The drawing under review shows one solid part. Ordinate dimensions are in mm from its lowest x, y, z. Coordinates: 2 decimals unless noted, no trailing zeros. Loops run counter-clockwise (first coordinate to the right, second up) from the corner with the lowest first, then second, coordinate; pieces in that order, holes last. Notation, with made-up numbers: M -12,-38 L 8,-38 A8 cw 8,-29 Z; hole C 83.5,30.25 d2. An arc over 180 degrees is marked long. Use one line per item in the form item = value.
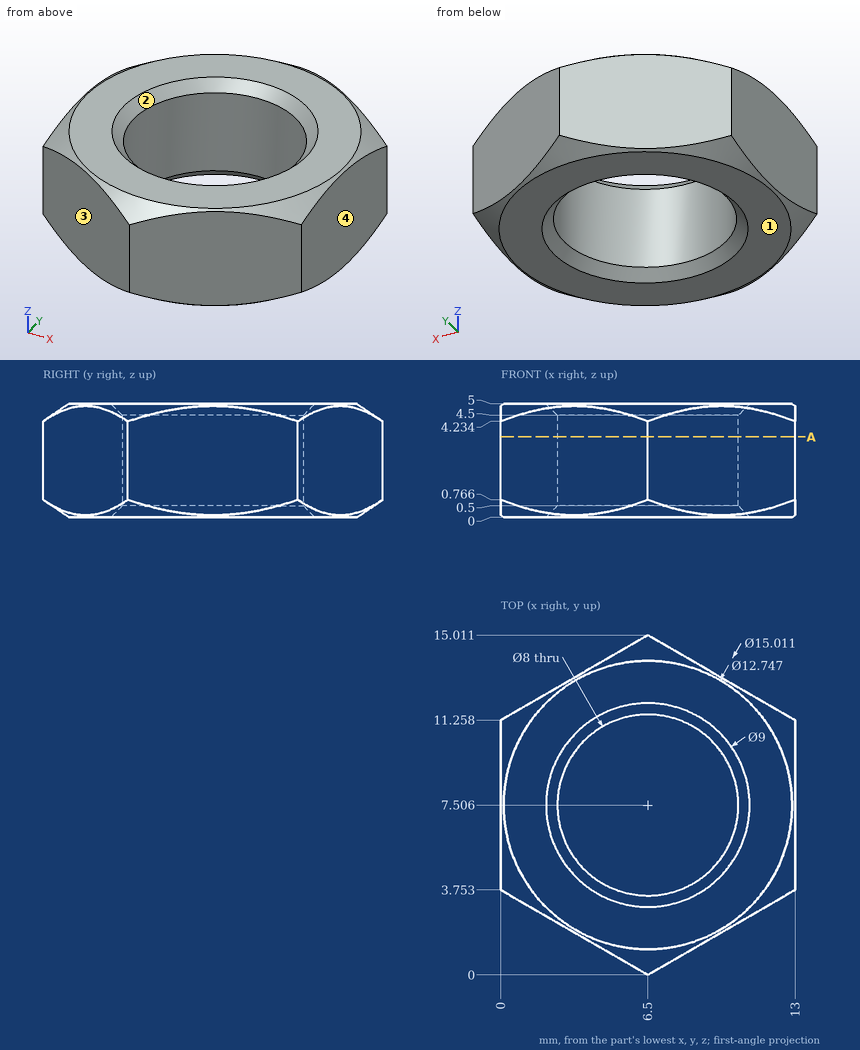
1. Wall thickness on line 1 along X through (y, z) = (10.5, 0.6); line 2 along X through (y, z) = (4, 3) (1 decimal); line 3 along Y through (x, z) = (4.75, 1.05): over which ranges is each line inside the solid? List them lowest first. Write a range as from..to.
Computed values:
line_1 = 0..3.85, 9.15..13
line_2 = 0..4.6, 8.4..13
line_3 = 1.01..3.91, 11.1..14
2. Draft analysis for pull direction X (two halves, no side actions). For the marked faces 1, 2, 3 and 4, state which applies: +X half, -X half, draft (parallel to the pull), parting line (faces both ways), or undercut.
Computed values:
face_1 = draft
face_2 = undercut
face_3 = -X half
face_4 = +X half
3. Consider section A-A on z = 3.55. Write out the cut boundary in (x, y) (1 decimal).
Computed values:
outline = M 0,3.8 L 6.5,0 L 13,3.8 L 13,11.3 L 6.5,15 L 0,11.3 Z; hole C 6.5,7.5 d8
4. For pin 1 Ø1.5 at (x, z) = (2.5, 4) entering from +Y (1 decimal), flat-tipped, find the tip position at first contact; note if it passes through.
Computed values:
pin_1 = 13.1
